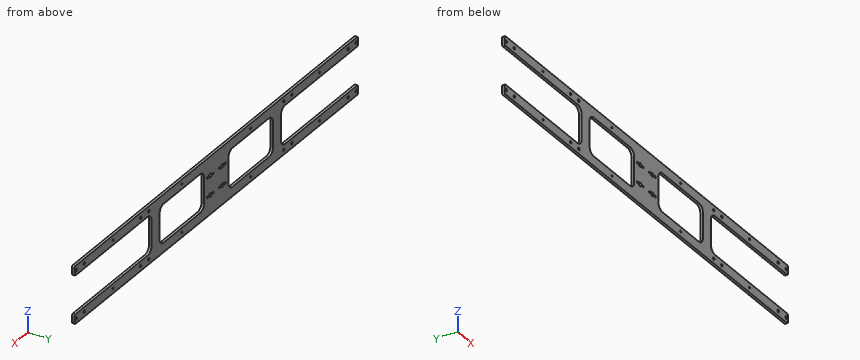
```python
from build123d import *

# Parameters (mm, degrees)
SKETCH_1_W                                   = 700
SKETCH_1_H                                   = 90
SKETCH_1_W_2                                 = 280
SKETCH_1_H_2                                 = 60
EXTRUDE_1_DEPTH                              = 4
SKETCH_2_W                                   = 190
SKETCH_2_H                                   = 60
CUT_EXTRUDE_1_DEPTH                          = 4
SKETCH_4_R                                   = 2
CUT_EXTRUDE_2_DEPTH                          = 15
MIRROR_2_AT_THE_SECOND_PLANE_COPY_1_SKET_R   = 2
MIRROR_2_AT_THE_SECOND_PLANE_COPY_1_DEPTH    = 15
SKETCH_5_W                                   = 60
SKETCH_5_H                                   = 60
EXTRUDE_2_DEPTH                              = 4
SKETCH_6_R                                   = 1.5
CUT_EXTRUDE_3_DEPTH                          = 4
MIRROR_3_AT_THE_SECOND_PLANE_COPY_1_SKET_R   = 1.5
MIRROR_3_AT_THE_SECOND_PLANE_COPY_1_DEPTH    = 4
FILLET_1_R                                   = 2
MIRROR_6_DEPTH                               = 4
EXTRUDE_3_DEPTH                              = 4
MIRROR_9_AT_THE_SECOND_PLANE_COPY_1_DEPTH    = 4
SKETCH_8_R                                   = 3
SKETCH_8_R_2                                 = 1.5
CUT_EXTRUDE_4_DEPTH                          = 15
MIRROR_10_AT_THE_SECOND_PLANE_COPY_1_SKE_R   = 3
MIRROR_10_AT_THE_SECOND_PLANE_COPY_1_SKE_R_2 = 1.5
MIRROR_10_AT_THE_SECOND_PLANE_COPY_1_DEPTH   = 15


# Read off the part's stored shape, not the designer's step: 镜向6
with BuildPart() as part:
    # 草图1 → 凸台-拉伸1 (new body)
    with BuildSketch(Plane(origin=(0, 0, 0), x_dir=(1, 0, 0), z_dir=(0, 1, 0))):
        Rectangle(SKETCH_1_W, SKETCH_1_H)
        Rectangle(SKETCH_1_W_2, SKETCH_1_H_2, mode=Mode.SUBTRACT)
    extrude(amount=EXTRUDE_1_DEPTH)

    # 草图2 → 切除-拉伸1 (cut)
    with BuildSketch(Plane(origin=(0, 4, 0), x_dir=(1, 0, 0), z_dir=(0, 1, 0))):
        with Locations((-255, 0)):
            Rectangle(SKETCH_2_W, SKETCH_2_H)
    cut_extrude_1 = extrude(amount=-CUT_EXTRUDE_1_DEPTH, mode=Mode.SUBTRACT)

    # 镜向1: 切除-拉伸1 across plane
    add(cut_extrude_1.mirror(Plane(origin=(0, 0, 0), x_dir=(0, 0, 1), z_dir=(1, 0, 0))), mode=Mode.SUBTRACT)

    # 草图4 → 切除-拉伸2 (cut)
    with BuildSketch(Plane(origin=(0, 4, 0), x_dir=(1, 0, 0), z_dir=(0, 1, 0))):
        with Locations(Location((-187, 37.5, 0), (0, 0, 270))):
            Circle(SKETCH_4_R)
        with Locations(Location((-167, 37.5, 0), (0, 0, 270))):
            Circle(SKETCH_4_R)
        with Locations(Location((-346, 37.5, 0), (0, 0, 270))):
            Circle(SKETCH_4_R)
        with Locations(Location((-326, 37.5, 0), (0, 0, 270))):
            Circle(SKETCH_4_R)
    cut_extrude_2 = extrude(amount=-CUT_EXTRUDE_2_DEPTH, mode=Mode.SUBTRACT)

    # 镜向2: 切除-拉伸2 across plane
    add(cut_extrude_2.mirror(Plane(origin=(0, 0, 0), x_dir=(0, 0, 1), z_dir=(1, 0, 0))), mode=Mode.SUBTRACT)

    # 镜向2 at the second plane: 切除-拉伸2 across plane
    add(cut_extrude_2.mirror(Plane.XY), mode=Mode.SUBTRACT)

    # 镜向2 at the second plane copy 1 sket → 镜向2 at the second plane copy 1 (cut)
    with BuildSketch(Plane(origin=(0, 4, 0), x_dir=(-1, 0, 0), z_dir=(0, 1, 0))):
        with Locations(Location((-187, 37.5, 0), (0, 0, 270))):
            Circle(MIRROR_2_AT_THE_SECOND_PLANE_COPY_1_SKET_R)
        with Locations(Location((-167, 37.5, 0), (0, 0, 270))):
            Circle(MIRROR_2_AT_THE_SECOND_PLANE_COPY_1_SKET_R)
        with Locations(Location((-346, 37.5, 0), (0, 0, 270))):
            Circle(MIRROR_2_AT_THE_SECOND_PLANE_COPY_1_SKET_R)
        with Locations(Location((-326, 37.5, 0), (0, 0, 270))):
            Circle(MIRROR_2_AT_THE_SECOND_PLANE_COPY_1_SKET_R)
    extrude(amount=-MIRROR_2_AT_THE_SECOND_PLANE_COPY_1_DEPTH, mode=Mode.SUBTRACT)

    # 草图5 → 凸台-拉伸2 (add)
    with BuildSketch(Plane(origin=(0, 4, 0), x_dir=(1, 0, 0), z_dir=(0, 1, 0))):
        Rectangle(SKETCH_5_W, SKETCH_5_H)
    extrude(amount=-EXTRUDE_2_DEPTH)

    # 草图6 → 切除-拉伸3 (cut)
    with BuildSketch(Plane(origin=(0, 4, 0), x_dir=(1, 0, 0), z_dir=(0, 1, 0))):
        with Locations(Location((-255, 37.5, 0), (0, 0, 270))):
            Circle(SKETCH_6_R)
        with Locations(Location((-85, 37.5, 0), (0, 0, 270))):
            Circle(SKETCH_6_R)
    cut_extrude_3 = extrude(amount=-CUT_EXTRUDE_3_DEPTH, mode=Mode.SUBTRACT)

    # 镜向3: 切除-拉伸3 across plane
    add(cut_extrude_3.mirror(Plane.XY), mode=Mode.SUBTRACT)

    # 镜向3 at the second plane: 切除-拉伸3 across plane
    add(cut_extrude_3.mirror(Plane(origin=(0, 0, 0), x_dir=(0, 0, 1), z_dir=(1, 0, 0))), mode=Mode.SUBTRACT)

    # 镜向3 at the second plane copy 1 sket → 镜向3 at the second plane copy 1 (cut)
    with BuildSketch(Plane(origin=(0, 4, 0), x_dir=(-1, 0, 0), z_dir=(0, 1, 0))):
        with Locations(Location((-255, 37.5, 0), (0, 0, 270))):
            Circle(MIRROR_3_AT_THE_SECOND_PLANE_COPY_1_SKET_R)
        with Locations(Location((-85, 37.5, 0), (0, 0, 270))):
            Circle(MIRROR_3_AT_THE_SECOND_PLANE_COPY_1_SKET_R)
    extrude(amount=-MIRROR_3_AT_THE_SECOND_PLANE_COPY_1_DEPTH, mode=Mode.SUBTRACT)

    # 圆角1
    fillet_1_edges = [part.edges().sort_by_distance(p)[0] for p in [
        (-350, 2, -30),
        (-350, 2, -45),
    ]]
    fillet(fillet_1_edges, radius=FILLET_1_R)

    # 镜向6 outline → 镜向6 (cut)
    with BuildSketch(Plane(origin=(0, 0, 0), x_dir=(1, 0, 0), z_dir=(0, 1, 0))):
        with BuildLine():
            Line((350, 45), (348, 45))
            ThreePointArc((348, 45), (349.414213562, 44.414213562), (350, 43))
            Line((350, 43), (350, 45))
        make_face()
        with BuildLine():
            Line((350, 30), (350, 32))
            ThreePointArc((350, 32), (349.414213562, 30.585786438), (348, 30))
            Line((348, 30), (350, 30))
        make_face()
        with BuildLine():
            Line((-350, -45), (-348, -45))
            ThreePointArc((-348, -45), (-349.414213562, -44.414213562), (-350, -43))
            Line((-350, -43), (-350, -45))
        make_face()
        with BuildLine():
            ThreePointArc((348, -30), (349.414213562, -30.585786438), (350, -32))
            Line((350, -32), (350, -30))
            Line((350, -30), (348, -30))
        make_face()
        with BuildLine():
            ThreePointArc((350, -43), (349.414213562, -44.414213562), (348, -45))
            Line((348, -45), (350, -45))
            Line((350, -45), (350, -43))
        make_face()
        with BuildLine():
            Line((-350, -30), (-350, -32))
            ThreePointArc((-350, -32), (-349.414213562, -30.585786438), (-348, -30))
            Line((-348, -30), (-350, -30))
        make_face()
    extrude(amount=MIRROR_6_DEPTH, mode=Mode.SUBTRACT)

    # 草图7 → 凸台-拉伸3 (add)
    with BuildSketch(Plane(origin=(0, 4, 0), x_dir=(1, 0, 0), z_dir=(0, 1, 0))):
        with BuildLine():
            Line((-170, 30), (-160, 30))
            Line((-160, 30), (-160, 20))
            ThreePointArc((-160, 20), (-162.928932188, 27.071067812), (-170, 30))
        make_face()
        with BuildLine():
            Line((-140, 20), (-140, 30))
            Line((-140, 30), (-130, 30))
            ThreePointArc((-130, 30), (-137.071067812, 27.071067812), (-140, 20))
        make_face()
        with BuildLine():
            Line((-40, 30), (-30, 30))
            Line((-30, 30), (-30, 20))
            ThreePointArc((-30, 20), (-32.928932188, 27.071067812), (-40, 30))
        make_face()
    extrude_3 = extrude(amount=-EXTRUDE_3_DEPTH)

    # 镜向9: 凸台-拉伸3 across plane
    add(extrude_3.mirror(Plane(origin=(0, 0, 0), x_dir=(0, 0, 1), z_dir=(1, 0, 0))))

    # 镜向9 at the second plane: 凸台-拉伸3 across plane
    add(extrude_3.mirror(Plane.XY))

    # 镜向9 at the second plane copy 1 sket → 镜向9 at the second plane copy 1 (add)
    with BuildSketch(Plane(origin=(0, 4, 0), x_dir=(-1, 0, 0), z_dir=(0, 1, 0))):
        with BuildLine():
            Line((-170, 30), (-160, 30))
            Line((-160, 30), (-160, 20))
            ThreePointArc((-160, 20), (-162.928932188, 27.071067812), (-170, 30))
        make_face()
        with BuildLine():
            Line((-140, 20), (-140, 30))
            Line((-140, 30), (-130, 30))
            ThreePointArc((-130, 30), (-137.071067812, 27.071067812), (-140, 20))
        make_face()
        with BuildLine():
            Line((-40, 30), (-30, 30))
            Line((-30, 30), (-30, 20))
            ThreePointArc((-30, 20), (-32.928932188, 27.071067812), (-40, 30))
        make_face()
    extrude(amount=-MIRROR_9_AT_THE_SECOND_PLANE_COPY_1_DEPTH)

    # 草图8 → 切除-拉伸4 (cut)
    with BuildSketch(Plane(origin=(0, 4, 0), x_dir=(1, 0, 0), z_dir=(0, 1, 0))):
        with Locations(Location((-15, 15, 0), (0, 0, 270))):
            Circle(SKETCH_8_R)
        with Locations(Location((-22, 15, 0), (0, 0, 270))):
            Circle(SKETCH_8_R_2)
        with Locations(Location((-8, 15, 0), (0, 0, 270))):
            Circle(SKETCH_8_R_2)
    cut_extrude_4 = extrude(amount=-CUT_EXTRUDE_4_DEPTH, mode=Mode.SUBTRACT)

    # 镜向10: 切除-拉伸4 across plane
    add(cut_extrude_4.mirror(Plane.XY), mode=Mode.SUBTRACT)

    # 镜向10 at the second plane: 切除-拉伸4 across plane
    add(cut_extrude_4.mirror(Plane(origin=(0, 0, 0), x_dir=(0, 0, 1), z_dir=(1, 0, 0))), mode=Mode.SUBTRACT)

    # 镜向10 at the second plane copy 1 ske → 镜向10 at the second plane copy 1 (cut)
    with BuildSketch(Plane(origin=(0, 4, 0), x_dir=(-1, 0, 0), z_dir=(0, 1, 0))):
        with Locations(Location((-15, 15, 0), (0, 0, 270))):
            Circle(MIRROR_10_AT_THE_SECOND_PLANE_COPY_1_SKE_R)
        with Locations(Location((-22, 15, 0), (0, 0, 270))):
            Circle(MIRROR_10_AT_THE_SECOND_PLANE_COPY_1_SKE_R_2)
        with Locations(Location((-8, 15, 0), (0, 0, 270))):
            Circle(MIRROR_10_AT_THE_SECOND_PLANE_COPY_1_SKE_R_2)
    extrude(amount=-MIRROR_10_AT_THE_SECOND_PLANE_COPY_1_DEPTH, mode=Mode.SUBTRACT)


solid = part.part
```
Source: CAD feature listing. Evaluate the final solid. Frame: model axes, mm. Round coordinates to 2 decimals unless told otherwise and drop trailing zeros. Order: outer loops, then holes, each group sorted by start corner. A loop starts at its lowest first (then second) coordinate and runs counter-clockwise, first axis right, second up. Notation, with made-up numbers: (12, 11) -> (34, 11) arc R22 ccw to (34, 17) -> close; hole circle Ø3 at (52, 45). An arc over 180 degrees is marked (long way). Use CSV: the item, a comma, the result in double quotes.
(1) Section A-A on x = -265. Return the cut outline in (y, z), and give its area (3 significant figures).
Report:
outline,"(0, -45) -> (4, -45) -> (4, -30) -> (0, -30) -> close; (0, 30) -> (4, 30) -> (4, 45) -> (0, 45) -> close"
area,"120 mm^2"
(2) Section B-B on y = 1.65. Count the separate pieces of the cut face and the enclosed holes in it, and give its area (3 significant figures).
Report:
separate pieces,"1"
enclosed holes,"38"
area,"26,800 mm^2"
(3) First-contact query: pin 1 Ø2 at (y, z) = (2.5, 6) entering from -X. Flat tip, straight axial feed; report the tip coordinate or a pass-through.
Report:
pin 1,"x = -160"
(4) Ray query, L1, parallel to Z at x = -187, y = 2.3; L2, parallel to Z at x = -279, y = 1.4; L3, parallel to Z at x = 22, y = 2.8. Return the intervals inside material, ascending.
Report:
L1,"-45 to -39.5, -35.5 to -30, 30 to 35.5, 39.5 to 45"
L2,"-45 to -30, 30 to 45"
L3,"-45 to -16.5, -13.5 to 13.5, 16.5 to 45"
